Part model, mm, in its own coordinate system. A direction names the side the tool comes from. Give positions to 0.01 mm unless a question says otherwise; leave off trailing zeros. Write each loop counter-clockwise with the first axis right and the second up, starting at its lowest first coordinate (ties: lowest second). Pieces come first, ordered by that corner, then holes. Notation, with made-up numbers: M 15,68 L 68,68 A21 ccw 68,81 Z; hole C -36.5,63.25 d11. An arc over 180 degrees is marked long. Answer as CSV lines item,"result". Start each with the question number.
1) Slice it at A-A, the plane y = 36. Give the cut face in (x, z).
2) Wall check: line 1 along Y through (x, z) = (0, 2.2); line 2 along Y through (x, z) = (0, 2.15); line 3 along Y through (x, z) = (1.5, 2.85). Give the ranges that are in metal, low to high. Write a range as from..to.
3) Tool access for faces 4 (the cylindrical face through (0.03, 22.74, 4.48)), 5 (the flat face through (8.14, 9.5, 1.99)), 6 (the flat face through (7.074, 29.839, 1.994)), 7 (the cylindrical face through (6.414, 29.555, 0.456)), 8 (the cylindrical face through (-11.96, -3.64, 3.52)): list every direction of +Z, -Z, +X, -X, +Y, -Y with a clear straight run to the whole face (end or side of a thin tool).
4) Mould opens along Y. For faces 1 (the flat face through (-7.074, 29.839, 1.994)), 2 (the flat face through (-2, 16, 0)), 3 (the cylindrical face through (-16.04, -17.02, 2.01)) say: pulls with the +Y half, pulls with the -Y half, needs draft (parallel to the pull), parting line crosses it, or undercut.
5) Slice it at B-B, the plane x = 0. Give the number of separate pieces and of enclosed holes in the cut face, plus the area to 3 significant figures.
6) Pin check, flat tips, straight feed: pin 1 Ø9 at (x, y) = (0, 36) entering from +Z; pin 2 Ø2 at (x, z) = (6.5, 0.5) entering from -Y; pin 3 Ø1.5 at (x, z) = (1, 4) entering from -Y; pin 4 Ø4 at (x, y) = (-2, 14) entering from +Z. Stop position of each tip, or through.
Autodesk Fusion 360 part; units mm, degrees
sketch "Sketch1" plane through (0, 0, 0) normal (0, 0, 1) x (1, 0, 0)
  line L0 (11.5, 12.5) -> (-11.5, 12.5)
  line L1 (-11.5, 12.5) -> (-11.5, -12.5)
  line L2 (-11.5, -12.5) -> (11.5, -12.5)
  line L3 (11.5, -12.5) -> (11.5, 12.5)
  line L4 (11.5, 12.5) -> (-11.5, -12.5) construction
  line L5 (-11.5, 12.5) -> (11.5, -12.5) construction
  line L6 (0, 38) -> (0, -20) construction
  line L7 (0, 27.5) -> (-6, 27.5)
  line L8 (16.5, -17.5) -> (16.5, 17.5)
  line L9 (16.5, 17.5) -> (-16.5, 17.5)
  line L10 (-16.5, 17.5) -> (-16.5, -17.5)
  line L11 (-16.5, -17.5) -> (16.5, -17.5)
  line L12 (-6, 27.5) -> (-16.5, 15.8333)
  line L13 (0, 27.5) -> (6, 27.5)
  line L14 (6, 27.5) -> (16.5, 15.8333)
  line L15 (-4.8766, 12.5) -> (-11.5, 6.4065)
  line L16 (4.8766, 12.5) -> (11.5, 6.4065)
  circle A0 centre (0, 36) radius 5
  circle A1 centre (0, 36) radius 9
  line L17 (0, 24.036) -> (-17, 24.036) construction
  line L18 (-6, 27.5) -> (-8.1787, 32.2438)
  line L19 (6, 27.5) -> (8.1787, 32.2438)
  point P0 (0, 24.036)
  dimension "d1" = 23
  dimension "d2" = 25
  dimension "d7" = 40
  dimension "d8" = 5
  dimension "d9" = 36.536
  dimension "d10" = 9
  dimension "d11" = 10
  dimension "d12" = 4
extrude "Extrude1" add sketch "Sketch1" along normal blind 4 contours L0 L3 L16 | L0 L1 L15 | L7 L13 A1 | L7 L13 A1 | L7 L9 L12 L13 L14 A1 | L7 A1 L18 | L13 A1 L19 | L8 L9 L10 L11 L12 L14
ref_plane "WorkPlane1" through (-8.5, 24.036, 0) normal (0, -0.7071, 0.7071) x (-1, 0, 0)
sketch "Sketch2" plane through (-8.5, 24.036, 0) normal (0, -0.7071, 0.7071) x (-1, 0, 0)
  circle A0 centre (-8.5, 0) radius 1.2
  circle A1 centre (-8.5, 0) radius 2.25
  circle A2 centre (-8.5, 0) radius 4
  point P0 (-8.5, 0)
  dimension "d16" = 2.4
  dimension "d17" = 4.5
  dimension "d18" = 8
extrude "Extrude2" cut sketch "Sketch2" along normal through all and the other way blind 7.753 contours A0
ref_plane "WorkPlane2" through (0, 20.854, 3.182) normal (0, -0.7071, 0.7071) x (-1, 0, 0)
sketch "Sketch3" plane through (0, 20.854, 3.182) normal (0, -0.7071, 0.7071) x (-1, 0, 0)
  circle A0 centre (0, 0) radius 1.2
  circle A1 centre (0, 0) radius 2.25
  circle A2 centre (0, 0) radius 4
extrude "Extrude4" cut sketch "Sketch3" along normal blind 10.1125 contours A1
extrude "Extrude6" add sketch "Sketch3" against normal blind 1.187 contours A1
fillet "Fillet1" radius 1.6 31 edges at (0, 45, 4) (-7.0893, 29.8719, 4) (7.0893, 29.8719, 4) (-4.6616, 37.8081, 4) (-4.6616, 37.8081, 0) (0, 45, 0) (-7.0893, 29.8719, 0) (7.0893, 29.8719, 0) (-11.25, 21.6667, 4) (-16.5, -0.8333, 4) (-16.5, -0.8333, 0) (0, -17.5, 4) (0, -17.5, 0) (16.5, -0.8333, 4) (16.5, -0.8333, 0) (-8.1883, 9.4532, 4) (0, 12.5, 4) (-11.5, -3.0468, 4) (0, -12.5, 4) (11.5, -3.0468, 4) (8.1883, 9.4532, 4) (11.5, -3.0468, 0) (0, -12.5, 0) (-11.5, -3.0468, 0) (0, 12.5, 0) (-8.1883, 9.4532, 0) (8.1883, 9.4532, 0) (11.25, 21.6667, 4) (11.25, 21.6667, 0) (16.5, -17.5, 2) (-16.5, -17.5, 2)
Found:
1,outline,"M -9,1.6 A1.6 ccw -7.4,0 L -6.6,0 A1.6 ccw -5,1.6 L -5,2.4 A1.6 ccw -6.6,4 L -7.4,4 A1.6 ccw -9,2.4 Z; M 5,1.6 A1.6 ccw 6.6,0 L 7.4,0 A1.6 ccw 9,1.6 L 9,2.4 A1.6 ccw 7.4,4 L 6.6,4 A1.6 ccw 5,2.4 Z"
2,line 1,"-17.5..-12.5, 12.5..18.65, 19.87..20.14, 23.53..31, 41..45"
2,line 2,"-17.5..-12.5, 12.5..18.7, 19.82..20.19, 23.58..31, 41..45"
2,line 3,"-17.44..-12.56, 12.56..18.81, 20.52..31.16, 40.84..44.81"
3,face 4,"+Z, +Y"
3,face 5,"+Z, -Z"
3,face 6,"+Z, -Z, +X"
3,face 7,"-Z, +X"
3,face 8,"+Z"
4,face 1,"undercut"
4,face 2,"needs draft"
4,face 3,"pulls with the -Y half"
5,separate pieces,"4"
5,enclosed holes,"0"
5,area,"87.4 mm²"
6,pin 1,"through"
6,pin 2,"y = -17.5"
6,pin 3,"y = -17.26"
6,pin 4,"z = 4"
